from build123d import *

# Parameters (mm, degrees)
F1_DEPTH = 25


# Not quite as in the source:
# - a feature names something its author has since deleted; it is built from what else it names


with BuildPart() as f1:
    # F0 (on Top) → F1 (new body)
    with BuildSketch(Plane.XY):
        with BuildLine():
            ThreePointArc((1, 15.3674981698), (11.2374374303, 10.5299572649), (15.4, 0))
            ThreePointArc((15.4, 0), (-10.5299572649, -11.2374374303), (-1, 15.3674981698))
            Line((-1, 15.3674981698), (-1, 19.9749843554))
            ThreePointArc((-1, 19.9749843554), (-4.5745212177, 19.4698165279), (-8, 18.3303027798))
            ThreePointArc((-8, 18.3303027798), (-10.9544511501, -16.7332005307), (20, 0))
            ThreePointArc((20, 0), (16.7332005307, 10.9544511501), (8, 18.3303027798))
            ThreePointArc((8, 18.3303027798), (4.5745212177, 19.4698165279), (1, 19.9749843554))
            Line((1, 19.9749843554), (1, 15.3674981698))
        make_face()
        with BuildLine():
            Line((1, 28.3303027798), (1, 19.9749843554))
            ThreePointArc((1, 19.9749843554), (4.5745212177, 19.4698165279), (8, 18.3303027798))
            Line((8, 18.3303027798), (8, 28.3303027798))
            Line((8, 28.3303027798), (1, 28.3303027798))
        make_face()
        with BuildLine():
            ThreePointArc((-8, 18.3303027798), (-4.5745212177, 19.4698165279), (-1, 19.9749843554))
            Line((-1, 19.9749843554), (-1, 28.3303027798))
            Line((-1, 28.3303027798), (-8, 28.3303027798))
            Line((-8, 28.3303027798), (-8, 18.3303027798))
        make_face()
    extrude(amount=F1_DEPTH)


solid = f1.part
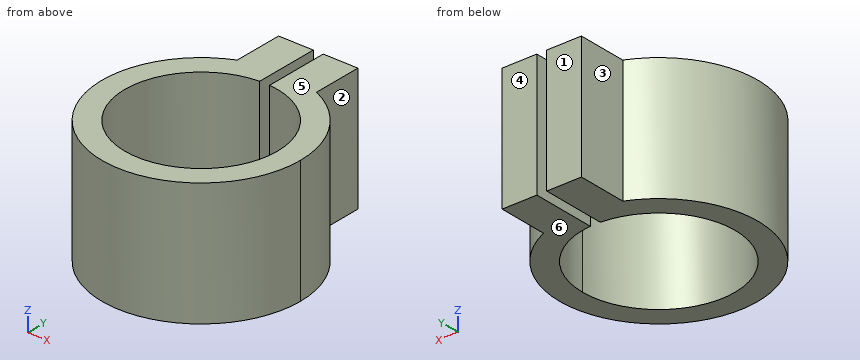
Read the model definition and answer for the solid it produces. Units are mm, in the model's axes. Face numbers are marked on the shaded views. A direction names the side the tool comes from. Coordinates: 2 decimals unless noted, no trailing zeros. Write each loop counter-clockwise with the first axis right and the second up, starting at its lowest first coordinate (ties: lowest second). Pieces come first, ordered by that corner, then holes. Notation, with made-up numbers: (86.25, 29.25) - (138.25, 29.25) arc R19 cw to (138.25, 61.25) - close; hole circle Ø9 at (42.25, 7). An arc over 180 degrees is marked (long way). One line per question, with ' | ' between items.
Q1. Determine the mould class of the marked faces 4, 5 and 6 for opening direction Z: +Z half, -Z half, draft (parallel to the pull), parting line (faces both ways), or undercut.
Result set:
face 4: draft | face 5: +Z half | face 6: -Z half
Q2. Find section B-B, the plane y = 1.5. Write down the section's boundary in (x, z), plus the area to 3 significant figures.
Result set:
outline: (-19.94, 0) - (-15.33, 0) - (-15.33, 25) - (-19.94, 25) - close; (15.33, 0) - (19.94, 0) - (19.94, 25) - (15.33, 25) - close | area: 231 mm^2
Q3. Find section D-D, the plane x = 0. Write down the section's boundary in (y, z).
Result set:
outline: (-20, 0) - (-15.4, 0) - (-15.4, 25) - (-20, 25) - close
Q4. Consider L1, parallel to X at y = 20, z = 23.5; L2, parallel to Y at x = 0, z = 5.25; L3, parallel to Y at x = 2.5, z = 22.75. Determine where each line is inside the solid, lowest interval first. Write a range as [from, to].
Result set:
L1: [-8, -1], [1, 8] | L2: [-20, -15.4] | L3: [-19.84, -15.2], [15.2, 28.33]
Q5. Find section A-A, the plane x = -12. Write down the section's boundary in (y, z).
Result set:
outline: (-16, 0) - (-9.65, 0) - (-9.65, 25) - (-16, 25) - close; (9.65, 0) - (16, 0) - (16, 25) - (9.65, 25) - close
Q6. For the marked faces 1, 2 and 3, determine the directions among +Z, -Z, +X, -X, +Y, -Y from which every point of the face is accessible in a straight line to the end or side of a thin tool.
Result set:
face 1: +Z, -Z, +X, -X, +Y | face 2: +Z, -Z, +X, +Y | face 3: +Z, -Z, -X, +Y
Q7. Each of these flat-tipped pins is pushed along its axis until it touches: P1, Ø5, axis at y = 23.5, z = 7, coming from the +X side; P2, Ø10.5, axis at y = 23.5, z = 17.5, coming from the +X side; P3, Ø1, axis at x = 2.5, y = 23, coming from the -Z side; P4, Ø1.5, axis at y = 2.5, z = 8.5, coming from the +X side. Where does it stop, or does it pass through?
Result set:
P1: x = 8 | P2: x = 8.18 | P3: z = 0 | P4: x = 19.92
Q8. Find section C-C, the plane z = 22.5. Write down the section's boundary in (x, y).
Result set:
outline: (-8, 18.33) arc R20 ccw (long way) to (8, 18.33) - (8, 28.33) - (1, 28.33) - (1, 15.37) arc R15.4 cw (long way) to (-1, 15.37) - (-1, 28.33) - (-8, 28.33) - close
